Autodesk Inventor part; units mm, degrees
ref_plane "YZ Plane" through (0, 0, 0) normal (1, 0, 0) x (0, 1, 0)
ref_plane "XZ Plane" through (0, 0, 0) normal (0, 1, 0) x (-1, 0, 0)
ref_plane "XY Plane" through (0, 0, 0) normal (0, 0, 1) x (1, 0, 0)
sketch "Sketch1" plane through (0, 0, 0) normal (1, 0, 0) x (0, 1, 0)
  line L0 (0, 0) -> (609.6, 0)
  line L1 (609.6, 0) -> (609.6, -908.05)
  line L2 (609.6, -908.05) -> (0, -908.05)
  line L3 (0, -908.05) -> (0, 0)
  line L4 (127, 0) -> (127, -908.05)
  line L5 (609.6, 0) -> (127, -127)
  line L6 (609.6, -908.05) -> (127, -781.05)
  line L7 (609.6, -76.2) -> (127, -203.2)
  line L8 (609.6, -831.85) -> (127, -704.85)
  dimension "d0" = 609.6
  dimension "d1" = 908.05
  dimension "d2" = 127
  dimension "d3" = 127
  dimension "d4" = 127
  dimension "d6" = 76.2
  dimension "d7" = 76.2
extrude "Plate1" add sketch "Sketch1" along normal blind 3.048 contours L0 L4 L2 L3 | L0 L5 L4 | L1 L7 L4 L5 | L4 L6 L2 | L6 L4 L8 L1
sketch "Sketch2" plane through (0, 609.6, -905.002) normal (0, 0, -1) x (-1, 0, 0)
  line L0 (0, -609.6) -> (0, 0)
  line L1 (0, 0) -> (-50.8, 0)
  line L2 (-50.8, 0) -> (-50.8, -609.6)
  line L3 (-50.8, -609.6) -> (0, -609.6)
edge flange "Flange1" height 50.8 angle 90 thickness 3.048 bend radius 3.048 thickness toward (0, 0, -1) relief tear relief width 3.048 relief depth 1.524 edges at (3.048, 304.8, -908.05) wall of the first edge with corners at (0, 0, -905.002) (0, 609.6, -905.002) (50.8, 609.6, -905.002) (50.8, 0, -905.002)
bend "Bend1"
corner "Corner1"
sketch "Sketch3" plane through (47.752, 609.6, -908.05) normal (1, 0, 0) x (0, 1, 0)
  line L0 (-609.6, 0) -> (0, 0)
  line L1 (0, 0) -> (0, 939.8)
  line L2 (0, 939.8) -> (-609.6, 939.8)
  line L3 (-609.6, 939.8) -> (-609.6, 0)
edge flange "Flange2" height 939.8 angle 90 thickness 3.048 bend radius 3.048 thickness toward (1, 0, 0) relief tear relief width 3.048 relief depth 1.524 edges at (50.8, 304.8, -905.002) wall of the first edge with corners at (47.752, 0, -908.05) (47.752, 609.6, -908.05) (47.752, 609.6, 31.75) (47.752, 0, 31.75)
bend "Bend2"
corner "Corner2"
sketch "Sketch4" plane through (0, 0, 0) normal (-1, 0, 0) x (0, 0, 1)
  line L0 (-901.954, 609.6) -> (-901.954, 0)
  line L1 (0, 0) -> (-901.954, 0)
  line L2 (0, 609.6) -> (0, 0)
  line L3 (-76.2, 609.6) -> (0, 609.6)
  line L4 (-203.2, 127) -> (-76.2, 609.6)
  line L5 (-704.85, 127) -> (-203.2, 127)
  line L6 (-831.85, 609.6) -> (-704.85, 127)
  line L7 (-901.954, 609.6) -> (-831.85, 609.6)
  line L8 (-908.05, 0) -> (-908.05, 609.6)
  line L9 (-901.954, 609.6) -> (-908.05, 609.6)
  line L10 (-908.05, 0) -> (-901.954, 0)
  line L11 (-908.05, 0) -> (-908.05, 609.6)
  line L12 (-901.954, 0) -> (-908.05, 0)
  line L13 (-901.954, 609.6) -> (-901.954, 0)
  line L14 (-908.05, 609.6) -> (-901.954, 609.6)
extrude "Extrusion1" cut sketch "Sketch4" against normal blind 76.2 keep common part
sketch "Sketch5" plane through (0, 0, -3.048) normal (0, 0, 1) x (1, 0, 0)
  line L0 (0, 609.6) -> (0, 0)
  line L1 (0, 0) -> (44.704, 0)
  line L2 (44.704, 0) -> (44.704, 609.6)
  line L3 (44.704, 609.6) -> (0, 609.6)
edge flange "Flange3" height 44.704 angle 90 thickness 3.048 bend radius 3.048 thickness toward (0, 0, 1) relief tear relief width 3.048 relief depth 1.524 edges at (3.048, 304.8, 0) wall of the first edge with corners at (0, 609.6, -3.048) (0, 0, -3.048) (44.704, 0, -3.048) (44.704, 609.6, -3.048)
bend "Bend3"
corner "Corner3"
equation "\"d8\" = Thickness"
equation "\"d9\" = BendReliefWidth"
equation "\"d10\" = BendReliefDepth"
equation "\"d11\" = MinimumRemnant"
equation "\"d12\" = TransitionRadius"
equation "\"d15\" = BendRadius"
equation "\"d16\" = CornerReliefSize"
equation "\"d17\" = GapSize"
equation "\"d18\" = JacobiRadiusSize"
equation "\"d19\" = BendReliefWidth"
equation "\"d20\" = BendReliefDepth"
equation "\"d21\" = MinimumRemnant"
equation "\"d22\" = TransitionRadius"
equation "\"d25\" = BendRadius"
equation "\"d26\" = CornerReliefSize"
equation "\"d27\" = GapSize"
equation "\"d28\" = JacobiRadiusSize"
equation "\"d31\" = BendReliefWidth"
equation "\"d32\" = BendReliefDepth"
equation "\"d33\" = MinimumRemnant"
equation "\"d34\" = TransitionRadius"
equation "\"d37\" = BendRadius"
equation "\"d38\" = CornerReliefSize"
equation "\"d39\" = GapSize"
equation "\"d40\" = JacobiRadiusSize"
equation "\"BendRadius\" = Thickness"
equation "\"BendReliefWidth\" = Thickness"
equation "\"BendReliefDepth\" = 0.5 * Thickness"
equation "\"CornerReliefSize\" = 4 * Thickness"
equation "\"MinimumRemnant\" = 2 * Thickness"
equation "\"TransitionRadius\" = BendRadius"
equation "\"JacobiRadiusSize\" = BendRadius"
equation "\"GapSize\" = Thickness"
properties part number "Div_Big"
Model file for the job. Use its own axes, mm. A direction names the side the tool comes from. Give positions to 0.01 mm unless a question says otherwise; leave off trailing zeros. Order: outer loops, then holes, each group sorted by start corner. A loop starts at its lowest first (then second) coordinate and runs counter-clockwise, first axis right, second up.
1) Pin check, flat tips, straight feed: pin 1 (1 mm diameter, centred on x = 5.5, z = -207, fed in from +Y); pin 2 (2.5 mm diameter, centred on x = 49.5, z = -523.5, fed in from +Y); pin 3 (10 mm diameter, centred on x = 24, y = 508, fed in from +Z). Stop position of each tip, or through.
2) 3-axis set-ups, long thin cutter, end or side, ignore diameter. For faces 4 (the flat face through (25, 309, -905.002)), 5 (the flat face through (1.5, 371.68, -769.24)), 6 (the flat face through (50.8, 106, -445)), 7 (the flat face through (47.752, 106, -457)): which of +Z, -Z, +X, -X, +Y, -Y reach the whole face in a straight line?
3) Wall check: probe 1 along Z at (x, y) = (29.5, 335.5); probe 2 along X at (y, z) = (278.5, -834.5); probe 3 along Z at (x, y) = (4.5, 579). Give the ranges that are in metal, low to high.
4) Mould opens along Z. For faces 1 (the flat face through (26, 309, -908.05)), 2 (the flat face through (48, 0, -452)), 3 (the flat face through (3.048, 97, -448)) say: +Z half, -Z half, draft (parallel to the pull), parting line (faces both ways), or undercut.
5) Saw through at B-B, the plane z = -166.5. Write the cut outline in (x, y), then the cut area to 3 significant figures.
6) Saw through at A-A, the plane y = 146. Write the cut outline in (x, z).
7) Saw through at D-D, the plane y = 471.5. Write the cut outline in (x, z).
8) Saw through at C-C, the plane x = 21. Write the cut outline in (y, z).
Computed:
1. pin 1: passes through
1. pin 2: stops at y = 127
1. pin 3: stops at z = 0
2. face 4: +Y, -Y
2. face 5: +X, -X, +Y
2. face 6: +Z, -Z, +X, +Y, -Y
2. face 7: +Z, +Y, -Y
3. probe 1: z = -908.05 to -905, -3.05 to 0
3. probe 2: x = 0 to 3.05, 47.75 to 50.8
3. probe 3: z = -907.84 to -904.55, -3.5 to -0.21
4. face 1: -Z half
4. face 2: draft
4. face 3: undercut
5. outline: (0, 0) - (3.05, 0) - (3.05, 266.46) - (0, 266.46) - close; (47.75, 0) - (50.8, 0) - (50.8, 266.46) - (47.75, 266.46) - close
5. area: 1,620 mm2
6. outline: (0, -901.95) arc R6.1 ccw to (6.1, -908.05) - (44.7, -908.05) arc R6.1 ccw to (50.8, -901.95) - (50.8, -709.85) - (47.75, -709.85) - (47.75, -901.95) arc R3.05 cw to (44.7, -905) - (6.1, -905) arc R3.05 cw to (3.05, -901.95) - (3.05, -709.85) - (0, -709.85) - close; (0, -198.2) - (3.05, -198.2) - (3.05, -6.1) arc R3.05 cw to (6.1, -3.05) - (44.7, -3.05) - (44.7, 0) - (6.1, 0) arc R6.1 ccw to (0, -6.1) - close; (47.75, -198.2) - (50.8, -198.2) - (50.8, 0) - (47.75, 0) - close
7. outline: (0, -901.95) arc R6.1 ccw to (6.1, -908.05) - (44.7, -908.05) arc R6.1 ccw to (50.8, -901.95) - (50.8, -795.51) - (47.75, -795.51) - (47.75, -901.95) arc R3.05 cw to (44.7, -905) - (6.1, -905) arc R3.05 cw to (3.05, -901.95) - (3.05, -795.51) - (0, -795.51) - close; (0, -112.54) - (3.05, -112.54) - (3.05, -6.1) arc R3.05 cw to (6.1, -3.05) - (44.7, -3.05) - (44.7, 0) - (6.1, 0) arc R6.1 ccw to (0, -6.1) - close; (47.75, -112.54) - (50.8, -112.54) - (50.8, 0) - (47.75, 0) - close
8. outline: (0, -908.05) - (609.6, -908.05) - (609.6, -905) - (0, -905) - close; (0, -3.05) - (609.6, -3.05) - (609.6, 0) - (0, 0) - close
